For this review, take the finished solid that the model builds, in its own axes (mm). Give positions to 0.01 mm unless a question says otherwise; leave off trailing zeros. Loops run counter-clockwise (first coordinate to the right, second up) from the corner with the lowest first, then second, coordinate; pieces in that order, holes last. Notation, with made-up numbers: (48.25, 51) -> (77.25, 51) arc R24 ccw to (77.25, 82) -> close; hole circle Ø11 at (-11, 76). An arc over 180 degrees is marked (long way). One line per question, with ' | ' between items. Start each with the question number.
(1) Wall thickness on probe 1 along X at (y, z) = (-0.5, 0.9); probe 2 along X at (y, z) = (-57, 1.85); probe 3 along X at (y, z) = (-50.5, 3.4): over which ranges is each line inside the solid? List them lowest first.
(2) Insertion check: P1, Ø1.2, axis at y = -55.5, z = 1.5, coming from the -X side; P2, Ø1, axis at y = -62.5, z = 1, coming from the +X side; P3, Ø2, axis at x = 0, y = -45, coming from the -Z side; P4, Ø1.5, axis at x = -4.5, z = 1.5, coming from the +Y side. Each pin has a flat end and moves straight along its axis. Give the tip position at first contact, or say it passes through.
(3) Consider section C-C (x = -12). Write out the cut boundary in (y, z).
(4) Consider section D-D (x = -16.5). Write out the cut boundary in (y, z).
(5) Consider section A-A (y = -4.5). Write out the cut boundary in (x, z), and give its area (3 significant figures).
(6) Consider section B-B (z = 1.9). Write out the cut boundary in (x, y).
from build123d import *

# Parameters (mm, degrees)
F0_R     = 1.25
F1_DEPTH = 4
F2_R     = 5
F3_R     = 5
F4_R     = 5


# Not quite as in the source:
# - ends of sketch curves that miss each other by under 0.0002 mm in the source are joined


with BuildPart() as f1:
    # F0 (on Top) → F1 (new body)
    with BuildSketch(Plane.XY):
        with BuildLine():
            ThreePointArc((-20.6, 0), (-10.3, 10.3), (0, 0))
            ThreePointArc((0, 0), (-0.7054288039, -3.746225242), (-2.7250880706, -6.9793057865))
            Line((-2.7250880706, -6.9793057865), (-7.8691552748, -20.1539324679))
            ThreePointArc((-7.8691552748, -20.1539324679), (4.8894066362, -13.467439476), (10, 0))
            ThreePointArc((10, 0), (-10.3, 20.3), (-30.6, 0))
            ThreePointArc((-30.6, 0), (-25.6, 3.8602209978), (-20.6, 0))
        make_face()
        with BuildLine():
            ThreePointArc((-20.4505253001, -1.748381003), (-20.5625632907, -0.8773794529), (-20.6, 0))
            ThreePointArc((-20.6, 0), (-25.6, 3.8602209978), (-30.6, 0))
            ThreePointArc((-30.6, 0), (-30.526216971, -1.7292041645), (-30.3054042323, -3.4458382874))
            ThreePointArc((-30.3054042323, -3.4458382874), (-24.722708741, -6.4013107037), (-20.4505253001, -1.748381003))
        make_face()
        with BuildLine():
            ThreePointArc((10, 0), (4.8894066362, -13.467439476), (-7.8691552748, -20.1539324679))
            Line((-7.8691552748, -20.1539324679), (-13.5885840282, -34.8021350801))
            Line((-13.5885840282, -34.8021350801), (-13.5885840282, -74.6936649084))
            Line((-13.5885840282, -74.6936649084), (10.083315894, -74.6936649084))
            Line((10.083315894, -74.6936649084), (10, 0))
        make_face()
        with Locations((0, -57.5)):
            Circle(F0_R, mode=Mode.SUBTRACT)
        with Locations((0, -45)):
            Circle(F0_R, mode=Mode.SUBTRACT)
    extrude(amount=F1_DEPTH)

    # F2
    f2_edges = [f1.edges().sort_by_distance(p)[0] for p in [
        (-13.588584, -74.693665, 2),
    ]]
    fillet(f2_edges, radius=F2_R)

    # F3
    f3_edges = [f1.edges().sort_by_distance(p)[0] for p in [
        (10.083316, -74.693665, 2),
    ]]
    fillet(f3_edges, radius=F3_R)

    # F4
    f4_edges = [f1.edges().sort_by_distance(p)[0] for p in [
        (-13.588584, -34.802135, 2),
    ]]
    fillet(f4_edges, radius=F4_R)


solid = f1.part
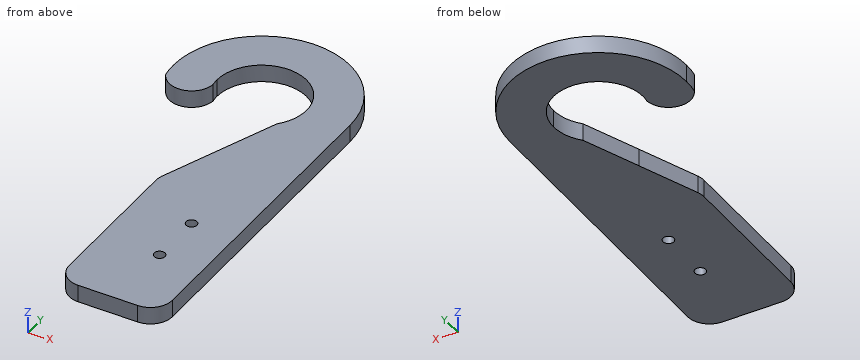
A:
1) probe 1: x = -30.59 to -20.59, -0.01 to 10 | probe 2: x = -13.59 to -1.15, 1.15 to 10.06 | probe 3: x = -13.59 to 10.06
2) P1: stops at x = -13.59 | P2: stops at x = 10.07 | P3: passes through | P4: stops at y = 19.66
3) outline: (-73.35, 0) -> (-30.73, 0) -> (-30.73, 4) -> (-73.35, 4) -> close; (10.16, 0) -> (20.23, 0) -> (20.23, 4) -> (10.16, 4) -> close
4) outline: (8.22, 0) -> (19.33, 0) -> (19.33, 4) -> (8.22, 4) -> close
5) outline: (-29.66, 0) -> (-21.54, 0) -> (-21.54, 4) -> (-29.66, 4) -> close; (-1.04, 0) -> (10.01, 0) -> (10.01, 4) -> (-1.04, 4) -> close | area: 76.7 mm^2
6) outline: (-30.31, -3.45) arc R5.17 ccw to (-20.45, -1.75) arc R10.3 cw (long way) to (-2.73, -6.98) -> (-13.25, -33.93) arc R5 ccw to (-13.59, -35.74) -> (-13.59, -69.69) arc R5 ccw to (-8.59, -74.69) -> (5.08, -74.69) arc R5 ccw to (10.08, -69.69) -> (10, 0) arc R20.3 ccw (long way) to start; hole circle Ø2.5 at (0, -57.5); hole circle Ø2.5 at (0, -45)
